from build123d import *

# Parameters (mm, degrees)
SKETCH1_R           = 3
BOSS_EXTRUDE1_DEPTH = 3.175


with BuildPart() as part:
    # Sketch1 → Boss-Extrude1 (new body)
    with BuildSketch(Plane(origin=(0, 0, 0), x_dir=(1, 0, 0), z_dir=(0, 1, 0))):
        with BuildLine():
            Line((-9.525, 0), (-9.525, -21.24))
            Line((-9.525, -21.24), (9.525, -21.24))
            Line((9.525, -21.24), (9.525, 0))
            ThreePointArc((9.525, 0), (0, 9.525), (-9.525, 0))
        make_face()
        Circle(SKETCH1_R, mode=Mode.SUBTRACT)
    extrude(amount=BOSS_EXTRUDE1_DEPTH)


solid = part.part
Here's how the part is built. I have some questions about the finished solid (model axes, mm). Coordinates: 2 decimals unless noted, no trailing zeros. Write each loop counter-clockwise with the first axis right and the second up, starting at its lowest first coordinate (ties: lowest second). Pieces come first, ordered by that corner, then holes. Notation, with made-up numbers: (-5.5, 18) - (53.5, 18) arc R10 cw to (53.5, 28) - close; hole circle Ø10 at (46.5, 15.25). An arc over 180 degrees is marked (long way). Use one line per item in the form item = value.
1) Suppose I cut it at B-B, the plane y = 2.5. Write out the boundary of the cut face in (x, z) (3 decimals).
Solved:
outline = (-9.525, 0) arc R9.525 ccw to (9.525, 0) - (9.525, 21.24) - (-9.525, 21.24) - close; hole circle Ø6 at (0, 0)
2) I need wall thicknesses on line 1 (Z direction, x = 0, y = 0.7) (3 decimals); line 2 (Z direction, x = -1.25, y = 2.25); line 3 (Z direction, x = -6, y = 0.4). Which ranges of each line are inside material? Lowest first, please.
Solved:
line_1 = -9.525 to -3, 3 to 21.24
line_2 = -9.44 to -2.73, 2.73 to 21.24
line_3 = -7.4 to 21.24
3) Suppose I cut it at C-C, the plane z = 1.5. Write out the boundary of the cut face in (x, y) (3 decimals).
Solved:
outline = (-9.525, 0) - (-2.598, 0) - (-2.598, 3.175) - (-9.525, 3.175) - close; (2.598, 0) - (9.525, 0) - (9.525, 3.175) - (2.598, 3.175) - close
4) Suppose I cut it at D-D, the plane x = -6.25. Write out the boundary of the cut face in (y, z) (3 decimals).
Solved:
outline = (0, -7.188) - (3.175, -7.188) - (3.175, 21.24) - (0, 21.24) - close
5) Suppose I cut it at A-A, the plane x = 0. Write out the boundary of the cut face in (y, z) (3 decimals).
Solved:
outline = (0, -9.525) - (3.175, -9.525) - (3.175, -3) - (0, -3) - close; (0, 3) - (3.175, 3) - (3.175, 21.24) - (0, 21.24) - close
6) Thinking about a two-plate mould opening in X: for faces 1 (the cylindrical face through (-3, 2, 0)), 2 (the flat face through (9.525, 2, 11)), 3 (the flat face through (-9.525, 2, 10)), 4 (the flat face through (0, 2, 21.24)), which applies, released by +X, released by -X, zero draft, split by the parting line, or undercut?
Solved:
face_1 = undercut
face_2 = released by +X
face_3 = released by -X
face_4 = zero draft
